Here's how the part is built. I have some questions about the finished solid (model axes, mm). Round coordinates to 2 decimals unless told otherwise and drop trailing zeros. Order: outer loops, then holes, each group sorted by start corner. A loop starts at its lowest first (then second) coordinate and runs counter-clockwise, first axis right, second up.
Autodesk Inventor part; units mm, degrees
ref_plane "YZ Plane" through (0, 0, 0) normal (1, 0, 0) x (0, 1, 0)
ref_plane "XZ Plane" through (0, 0, 0) normal (0, 1, 0) x (-1, 0, 0)
ref_plane "XY Plane" through (0, 0, 0) normal (0, 0, 1) x (1, 0, 0)
sketch "Szkic1" plane through (0, 0, 0) normal (0, 0, 1) x (1, 0, 0)
  line L0 (-9.5597, 36.3357) -> (54.4403, 36.3357)
  line L1 (54.4403, 36.3357) -> (54.4403, -9.7143)
  line L2 (54.4403, -9.7143) -> (-9.5597, -9.7143)
  line L3 (-9.5597, -9.7143) -> (-9.5597, 36.3357)
  point P0 (0, 0)
  point P1 (-4.0597, 26.7857)
  point P2 (26.9403, 26.7857)
  point P3 (-4.0597, -4.2143)
  point P4 (26.9403, -4.2143)
  point P5 (11.4403, 11.2857)
  point P6 (44.4403, 18.3357)
  point P7 (44.4403, -1.6893)
  dimension "d0" = 46.05
  dimension "d1" = 64
  dimension "d2" = 15.5
  dimension "d3" = 15.5
  dimension "d4" = 15.5
  dimension "d5" = 15.5
  dimension "d6" = 15.5
  dimension "d7" = 15.5
  dimension "d8" = 15.5
  dimension "d9" = 15.5
  dimension "d11" = 43
  dimension "d12" = 25.05
  dimension "d33" = 10
  dimension "d34" = 10
  dimension "d35" = 8.025
  dimension "d37" = 18
extrude "Wyciągnięcie proste1" add sketch "Szkic1" along normal blind 4
hole "Otwór1" at (11.4403, 11.2857, 0) direction (0, 0, 1) diameter 22.5 end through all
hole "Otwór2" at (26.9403, -4.2143, 0) at (-4.0597, -4.2143, 0) at (26.9403, 26.7857, 0) at (-4.0597, 26.7857, 0) direction (0, 0, 1) diameter 3 end through all
chamfer "Faza1" distance 2 angle 45 2 edges at (-9.5597, 36.3357, 2) (-9.5597, -9.7143, 2)
fillet "Zaokrąglenie1" radius 4 1 edges at (54.4403, -9.7143, 2)
hole "Otwór3" at (44.4403, 18.3357, 0) at (44.4403, -1.6893, 0) direction (0, 0, 1) diameter 5 end through all
properties part number "LC_ALU_4mm_Z_Axis_Motor_Mount"
1. If we section it at B-B, the plane x = 43.5: Write out the boundary of the cut face in (y, z).
Evaluation:
outline: (-9.71, 0) - (-4.01, 0) - (-4.01, 4) - (-9.71, 4) - close; (0.63, 0) - (16.02, 0) - (16.02, 4) - (0.63, 4) - close; (20.65, 0) - (36.34, 0) - (36.34, 4) - (20.65, 4) - close
2. I'm going to push a flat-ended pin straight in: P1, Ø2.5, axis at x = -4.06, y = 26.79, coming from the +Z side. Where does the tip first touch, or does it pass through?
Evaluation:
P1: passes through
3. If we mould it in two halves opening along X, with no side actions, what happens to faces 1 (the cylindrical face through (-3.147, -5.405, 2.028)), 2 (the cylindrical face through (25.453, -4.41, 2.028)), 3 (the flat face through (-8.546, -8.728, 2.028)), 4 (the cylindrical face through (53.24, -8.57, 2.03))? For each: released by +X, released by -X, zero draft, split by the parting line, or undercut.
Evaluation:
face 1: undercut
face 2: undercut
face 3: released by -X
face 4: released by +X
4. If we section it at A-A, the plane x = 1.5: Write out the boundary of the cut face in (y, z).
Evaluation:
outline: (-9.71, 0) - (6.02, 0) - (6.02, 4) - (-9.71, 4) - close; (16.55, 0) - (36.34, 0) - (36.34, 4) - (16.55, 4) - close
5. If we section it at D-D, the plane z = 3.1: Write out the boundary of the cut face in (x, y).
Evaluation:
outline: (-9.56, -7.71) - (-7.56, -9.71) - (50.44, -9.71) arc R4 ccw to (54.44, -5.71) - (54.44, 36.34) - (-7.56, 36.34) - (-9.56, 34.34) - close; hole circle Ø3 at (-4.06, -4.21); hole circle Ø3 at (-4.06, 26.79); hole circle Ø22.5 at (11.44, 11.29); hole circle Ø3 at (26.94, -4.21); hole circle Ø3 at (26.94, 26.79); hole circle Ø5 at (44.44, -1.69); hole circle Ø5 at (44.44, 18.34)
6. If we section it at C-C, the plane y = -1: Write out the boundary of the cut face in (x, z), and give its area (3 significant figures).
Evaluation:
outline: (-9.56, 0) - (42.04, 0) - (42.04, 4) - (-9.56, 4) - close; (46.84, 0) - (54.44, 0) - (54.44, 4) - (46.84, 4) - close
area: 237 mm2
7. I need wall thicknesses on probe 1 along X at (y, z) = (27, 2.55); probe 2 along X at (y, z) = (11, 3); probe 3 along Y at (x, z) = (-4, 1.8). Which ranges of each line are inside material? Lowest first, please.
Evaluation:
probe 1: x = -9.56 to -5.54, -2.58 to 25.46, 28.42 to 54.44
probe 2: x = -9.56 to 0.19, 22.69 to 54.44
probe 3: y = -9.71 to -5.71, -2.72 to 25.29, 28.28 to 36.34
